Autodesk Inventor part; units mm, degrees
ref_plane "YZ Plane" through (0, 0, 0) normal (1, 0, 0) x (0, 1, 0)
ref_plane "XZ Plane" through (0, 0, 0) normal (0, 1, 0) x (-1, 0, 0)
ref_plane "XY Plane" through (0, 0, 0) normal (0, 0, 1) x (1, 0, 0)
sketch "Sketch1" plane through (0, 0, 0) normal (0, 1, 0) x (-1, 0, 0)
  line L0 (0, 0) -> (60, 0)
  line L1 (60, 0) -> (60, -40)
  line L2 (60, -40) -> (0, -40)
  line L3 (0, -40) -> (0, 0)
  line L4 (50.9991, -13.6825) -> (46.57, -16.2397)
  line L5 (46.57, -16.2397) -> (42.1408, -13.6825)
  line L6 (42.1408, -13.6825) -> (42.1408, -8.5682)
  line L7 (42.1408, -8.5682) -> (46.57, -6.011)
  line L8 (46.57, -6.011) -> (50.9991, -8.5682)
  line L9 (50.9991, -8.5682) -> (50.9991, -13.6825)
  line L10 (50.6022, -31.0448) -> (46.57, -33.3728)
  line L11 (46.57, -33.3728) -> (42.5377, -31.0448)
  line L12 (42.5377, -31.0448) -> (42.5377, -26.3887)
  line L13 (42.5377, -26.3887) -> (46.57, -24.0607)
  line L14 (46.57, -24.0607) -> (50.6022, -26.3887)
  line L15 (50.6022, -26.3887) -> (50.6022, -31.0448)
  line L16 (46.57, 0) -> (46.57, -40) construction
  line L17 (60, -11.1253) -> (0, -11.1253) construction
  line L18 (0, -28.7167) -> (60, -28.7167) construction
  line L19 (31.3507, 0) -> (31.3507, -40) construction
  circle A0 centre (31.3507, -11.1253) radius 4
  circle A1 centre (31.3507, -28.7167) radius 5
  line L20 (18.6139, 0) -> (18.6139, -40) construction
  circle A2 centre (18.6139, -11.1253) radius 1.8986
  circle A3 centre (18.6139, -28.7167) radius 2.5527
  line L21 (8.1189, 0) -> (8.1189, -40) construction
  circle A4 centre (8.1189, -11.1253) radius 1.6319
  circle A5 centre (8.1189, -28.7167) radius 1.8987
  point P0 (46.57, -11.1253)
  point P1 (46.57, -28.7167)
  dimension "d0" = 60
  dimension "d1" = 40
  dimension "d2" = 8.8582
  dimension "d3" = 8.0645
  dimension "d4" = 8
  dimension "d5" = 10
  dimension "d6" = 3.7973
  dimension "d7" = 5.1054
  dimension "d8" = 3.2639
  dimension "d9" = 3.7973
  dimension "d23" = 9.3121
  dimension "d24" = 10.2286
extrude "Extrusion1" add sketch "Sketch1" along normal blind 10
properties part number "DimensionalCalibration"
Check sheet for the modelled part. Datum: model origin and axes. Units: mm. A direction names the side the tool comes from. Coordinates: 2 decimals unless noted, no trailing zeros. Write each loop counter-clockwise with the first axis right and the second up, starting at its lowest first coordinate (ties: lowest second). Pieces come first, ordered by that corner, then holes. Notation, with made-up numbers: (65.5, 45) - (81.5, 45) arc R14 cw to (81.5, 68) - close; hole circle Ø2 at (27, 28). An arc over 180 degrees is marked (long way). One line per question, with ' | ' between items.
Item 1: Sectioned sample at B-B on x = -49. Record the boundary of the cut face in (y, z).
Determined:
outline: (0, -40) - (10, -40) - (10, -31.97) - (0, -31.97) - close; (0, -25.46) - (10, -25.46) - (10, -14.84) - (0, -14.84) - close; (0, -7.41) - (10, -7.41) - (10, 0) - (0, 0) - close
Item 2: Mould release check, pull along X, two halves, no side actions. Record for faces 1 (the face through (0, 5, -20)), 2 (the face through (-30, 10, -20)), 3 (the face through (-50.999, 5, -11)): pulls with the +X half, pulls with the -X half, needs draft (parallel to the pull), parting line crosses it, or undercut.
Determined:
face 1: pulls with the +X half | face 2: needs draft | face 3: undercut
Item 3: Thickness scan on line 1 (X direction, y = 6.75, z = -28.5); line 2 (X direction, y = 1.25, z = -33); line 3 (X direction, y = 2.5, z = -10). Record the ranges inside material, lowest first. Write a range as [from, to].
Determined:
line 1: x = [-60, -50.6], [-42.54, -36.35], [-26.36, -21.16], [-16.07, -10.01], [-6.23, 0] | line 2: x = [-60, -47.22], [-45.92, -33.93], [-28.77, 0] | line 3: x = [-60, -51], [-42.14, -35.19], [-27.51, -20.14], [-17.08, -9.3], [-6.94, 0]
Item 4: Access from +Z, -Z, +X, -X, +Y, -Y to the whole of each face (thin tool, end or side, straight path). Record for faces 4 (the face through (-30, 5, -40)), 5 (the face through (-44.582, 4.93, -32.225)).
Determined:
face 4: -Z, +X, -X, +Y, -Y | face 5: +Y, -Y
Item 5: Sectioned sample at A-A on z = -25. Record the boundary of the cut face in (x, y), plus the area to 3 significant figures.
Determined:
outline: (-60, 0) - (-48.2, 0) - (-48.2, 10) - (-60, 10) - close; (-44.94, 0) - (-34.7, 0) - (-34.7, 10) - (-44.94, 10) - close; (-28.01, 0) - (0, 0) - (0, 10) - (-28.01, 10) - close | area: 501 mm2
Item 6: Sectioned sample at C-C on y = 8.5. Give the number of separate pieces and of enclosed holes in the cut face, plus the area to 3 significant figures.
Determined:
separate pieces: 1 | enclosed holes: 8 | area: 2,100 mm2
Item 7: Gauge pin test, flat end, axial feed: P1, Ø4.5, axis at x = -18.61, z = -28.72, coming from the -Y side. Record the tip position at first contact, or that the pin passes through.
Determined:
P1: passes through
Item 8: Sectioned sample at D-D on z = -10.5. Record the boundary of the cut face in (x, y), plus the area to 3 significant figures.
Determined:
outline: (-60, 0) - (-51, 0) - (-51, 10) - (-60, 10) - close; (-42.14, 0) - (-35.3, 0) - (-35.3, 10) - (-42.14, 10) - close; (-27.4, 0) - (-20.41, 0) - (-20.41, 10) - (-27.4, 10) - close; (-16.82, 0) - (-9.63, 0) - (-9.63, 10) - (-16.82, 10) - close; (-6.61, 0) - (0, 0) - (0, 10) - (-6.61, 10) - close | area: 366 mm2
